from build123d import *

# Parameters (mm, degrees)
F2_DEPTH  = 4
F3_R      = 3.8
F4_DEPTH  = 13
F5_R      = 3.8
F6_DEPTH  = 0.5
F6_TAPER  = -45
F7_R      = 4.3
F8_DEPTH  = 0.5
F8_TAPER  = 45
F9_W      = 1
F9_H      = 11
F10_DEPTH = 13
F11_R     = 4
F12_DEPTH = 3
F13_R     = 4
F14_DEPTH = 0.5
F14_TAPER = -45
F15_DEPTH = 0.5
F16_R     = 4.75
F16_R_2   = 4
F16_R_3   = 3.8
F17_DEPTH = 1
F18_W     = 11.6
F18_H     = 11.6
F19_DEPTH = 5


with BuildPart() as f2:
    # F1 (on Top) → F2 (new body)
    with BuildSketch(Plane.XY):
        with BuildLine():
            add(Edge.make_bspline(
                [(-62.9584054212, 12), (-50.9998563223, 0), (-9.8574829598, -7.14219171), (9.8574829598, -7.14219171), (50.9998563223, 0), (62.9584054212, 12)],
                knots=[0, 0, 0, 0, 0.3750382163, 0.6249617837, 1, 1, 1, 1], degree=3))
            ThreePointArc((-62.9584054212, 12), (-90.5016960105, 6.9783537313), (-76, -16.9705627485))
            Line((-76, -16.9705627485), (-68, -16.9705627485))
            Line((-68, -16.9705627485), (-68, -19.9705627485))
            Line((-68, -19.9705627485), (-60, -19.9705627485))
            Line((-60, -19.9705627485), (-60, -16.9705627485))
            Line((-60, -16.9705627485), (60, -16.9705627485))
            Line((60, -16.9705627485), (60, -19.9705627485))
            Line((60, -19.9705627485), (68, -19.9705627485))
            Line((68, -19.9705627485), (68, -16.9705627485))
            Line((68, -16.9705627485), (76, -16.9705627485))
            ThreePointArc((76, -16.9705627485), (90.5016960105, 6.9783537313), (62.9584054212, 12))
        make_face()
    extrude(amount=F2_DEPTH)

    # F3 (on face) → F4 (join)
    with BuildSketch(Plane.XY.offset(4)):
        with Locations((75, 0)):
            Circle(F3_R)
    extrude(amount=F4_DEPTH)

    # F5 (on face) → F6 (join)
    with BuildSketch(Plane.XY.offset(17)):
        with Locations((75, 0)):
            Circle(F5_R)
    extrude(amount=F6_DEPTH, taper=F6_TAPER)

    # F7 (on face) → F8 (join)
    with BuildSketch(Plane.XY.offset(17.5)):
        with Locations((75, 0)):
            Circle(F7_R)
    extrude(amount=F8_DEPTH, taper=F8_TAPER)

    # F9 (on face) → F10 (cut)
    with BuildSketch(Plane.XY.offset(18)):
        with Locations((75, 0)):
            Rectangle(F9_W, F9_H)
    extrude(amount=-F10_DEPTH, mode=Mode.SUBTRACT)

    # F11 (on face) → F12 (cut)
    with BuildSketch(Plane.XY.offset(4)):
        with Locations((-75, 0)):
            Circle(F11_R)
    extrude(amount=-F12_DEPTH, mode=Mode.SUBTRACT)

    # F13 (on face) → F14 (cut)
    with BuildSketch(Plane.XY.offset(1)):
        with Locations((-75, 0)):
            Circle(F13_R)
    extrude(amount=-F14_DEPTH, taper=F14_TAPER, mode=Mode.SUBTRACT)

    # F15 (cut): a face of the model
    f15_faces = [f2.faces().sort_by_distance(p)[0] for p in [
        (-75, 0, 0.5),
    ]]
    extrude(f15_faces, amount=-F15_DEPTH, mode=Mode.SUBTRACT)

    # F16 (on face) → F17 (join)
    with BuildSketch(Plane.XY.offset(4)):
        with Locations((-75, 0)):
            Circle(F16_R)
        with Locations((-75, 0)):
            Circle(F16_R_2, mode=Mode.SUBTRACT)
        with Locations((75, 0)):
            Circle(F16_R)
        with Locations((75, 0)):
            Circle(F16_R_3, mode=Mode.SUBTRACT)
    extrude(amount=F17_DEPTH)

    # F18 (on face) → F19 (cut)
    with BuildSketch(Plane.XY.offset(18)):
        with Locations((75, 0)):
            Rectangle(F18_W, F18_H)
        Polygon((71.2, 0), (71.2, 3.8), (78.8, 3.8), (78.8, -3.8), (71.2, -3.8), align=None, mode=Mode.SUBTRACT)
    extrude(amount=-F19_DEPTH, mode=Mode.SUBTRACT)


solid = f2.part
Can you work these out from the model? Positions are in its coordinate system, mm. A direction names the side the tool comes from. Coordinates: 2 decimals unless noted, no trailing zeros. Order: outer loops, then holes, each group sorted by start corner. A loop starts at its lowest first (then second) coordinate and runs counter-clockwise, first axis right, second up. Notation, with made-up numbers: (50, 83) -> (97, 83) arc R24 ccw to (97, 114) -> close; hole circle Ø5 at (-11, -4.5). An arc over 180 degrees is marked (long way). Use one line per item in the form item = value.
Q1. Which directions (+Z, -Z, +X, -X, +Y, -Y) give clear straight access to the entire face, cutting with the end or side of a thin tool? Please do faces 4 (the face through (72.062, 2.629, 17.142)), 5 (the face through (70.255, 0.209, 4.493)), 6 (the face through (72.46, -3.01, 17.14)).
From the geometry:
face_4 = -X, +Y
face_5 = +Z
face_6 = -X, -Y
Q2. We'd pull the mould along Z, two halves only. Please class faces 1 (the face through (77.938, -2.629, 17.142)), 2 (the face through (-64, -19.971, 2)), 3 (the face through (72.015, -2.565, 17.865)): released by +Z, released by -Z, zero draft, split by the parting line, or undercut.
From the geometry:
face_1 = undercut
face_2 = zero draft
face_3 = released by +Z
Q3. Imagine slicing it at A-A, the plane y = -8.5. List the corners of the cut face in (x, z) for me, then the cut area to 3 significant figures.
From the geometry:
outline = (-89.72, 0) -> (89.72, 0) -> (89.72, 4) -> (-89.72, 4) -> close
area = 718 mm²
Q4. I need wall thicknesses on L1, parallel to Y at x = -75, z = 0.3; L2, parallel to Y at x = -75, z = 1.95; L3, parallel to Z at x = -83.5, y = -9. Which ranges of each line are inside material? Lowest first, please.
From the geometry:
L1 = -16.97 to -4.5, 4.5 to 17
L2 = -16.97 to -4, 4 to 17
L3 = 0 to 4
Q5. Imagine slicing it at B-B, the plane x = 66. List the corners of the cut face in (y, z) for me, then the cut area to 3 significant figures.
From the geometry:
outline = (-19.97, 0) -> (14.42, 0) -> (14.42, 4) -> (-19.97, 4) -> close
area = 138 mm²
Q6. Will these pins go through, and if not, where does the flat tip stop? P1, Ø1, axis at x = 73.5, z = 17.5, coming from the +Y side; P2, Ø4.5, axis at x = 27.5, z = 2.5, coming from the -Y side; P3, Ø3, axis at x = -76.5, y = 0, coming from the +Z side (3 decimals); P4, Ø1.5, axis at y = -19, z = 1.5, coming from the +X side.
From the geometry:
P1 = 3.8
P2 = -16.97
P3 = through
P4 = 68
